from build123d import *

# Parameters (mm, degrees)
SKETCH_1_R          = 65
SKETCH_1_R_2        = 50.2
SKETCH_1_R_3        = 0.5
EXTRUDE_1_DEPTH     = 10
SKETCH_2_R          = 53
CUT_EXTRUDE_1_DEPTH = 8
CUT_EXTRUDE_START   = -8
SKETCH_9_R          = 65
SKETCH_9_R_2        = 55
CUT_EXTRUDE_2_DEPTH = 8
SKETCH_11_R         = 65
SKETCH_11_R_2       = 55
CUT_EXTRUDE_4_DEPTH = 15
SKETCH_12_R         = 53
CUT_EXTRUDE_6_DEPTH = 15
SKETCH_13_R         = 55
SKETCH_13_R_2       = 50.2
EXTRUDE_2_DEPTH     = 2
EXTRUDE_START       = -2
SKETCH_14_R         = 65
SKETCH_14_R_2       = 2.05
SKETCH_14_R_3       = 50.2
EXTRUDE_3_DEPTH     = 2


with BuildPart() as part:
    # 草图1 → 凸台-拉伸1 (new body)
    with BuildSketch(Plane.XY):
        Circle(SKETCH_1_R)
        Circle(SKETCH_1_R_2, mode=Mode.SUBTRACT)
        with Locations((0, 59)):
            Circle(SKETCH_1_R_3, mode=Mode.SUBTRACT)
        with Locations((29.5, 51.095498823)):
            Circle(SKETCH_1_R_3, mode=Mode.SUBTRACT)
        with Locations((51.095498823, 29.5)):
            Circle(SKETCH_1_R_3, mode=Mode.SUBTRACT)
        with Locations((59, 0)):
            Circle(SKETCH_1_R_3, mode=Mode.SUBTRACT)
        with Locations((51.095498823, -29.5)):
            Circle(SKETCH_1_R_3, mode=Mode.SUBTRACT)
        with Locations((29.5, -51.095498823)):
            Circle(SKETCH_1_R_3, mode=Mode.SUBTRACT)
        with Locations((0, -59)):
            Circle(SKETCH_1_R_3, mode=Mode.SUBTRACT)
        with Locations((-29.5, -51.095498823)):
            Circle(SKETCH_1_R_3, mode=Mode.SUBTRACT)
        with Locations((-51.095498823, -29.5)):
            Circle(SKETCH_1_R_3, mode=Mode.SUBTRACT)
        with Locations((-59, 0)):
            Circle(SKETCH_1_R_3, mode=Mode.SUBTRACT)
        with Locations((-51.095498823, 29.5)):
            Circle(SKETCH_1_R_3, mode=Mode.SUBTRACT)
        with Locations((-29.5, 51.095498823)):
            Circle(SKETCH_1_R_3, mode=Mode.SUBTRACT)
    extrude(amount=EXTRUDE_1_DEPTH)

    # 草图2 → 切除-拉伸1 (cut)
    with BuildSketch(Plane(origin=(0, 0, 0), x_dir=(-1, 0, 0), z_dir=(0, 0, -1))):
        Circle(SKETCH_2_R)
    extrude(amount=-CUT_EXTRUDE_1_DEPTH, mode=Mode.SUBTRACT)

    # 草图9 → 切除-拉伸2 (cut)
    with BuildSketch(Plane.XY.offset(10).offset(CUT_EXTRUDE_START)):
        Circle(SKETCH_9_R)
        Circle(SKETCH_9_R_2, mode=Mode.SUBTRACT)
    extrude(amount=CUT_EXTRUDE_2_DEPTH, mode=Mode.SUBTRACT)

    # 草图11 → 切除-拉伸4 (cut, symmetric)
    with BuildSketch(Plane.XY.offset(2)):
        Circle(SKETCH_11_R)
        Circle(SKETCH_11_R_2, mode=Mode.SUBTRACT)
    extrude(amount=CUT_EXTRUDE_4_DEPTH, both=True, mode=Mode.SUBTRACT)

    # 草图12 → 切除-拉伸6 (cut, symmetric)
    with BuildSketch(Plane(origin=(0, 0, 8), x_dir=(-1, 0, 0), z_dir=(0, 0, -1))):
        Circle(SKETCH_12_R)
    extrude(amount=CUT_EXTRUDE_6_DEPTH, both=True, mode=Mode.SUBTRACT)

    # 草图13 → 凸台-拉伸2 (add, symmetric)
    with BuildSketch(Plane(origin=(0, 0, 0), x_dir=(-1, 0, 0), z_dir=(0, 0, -1))):
        with Locations(Location((0, 0, 0), (0, 0, 180))):
            Circle(SKETCH_13_R)
        Circle(SKETCH_13_R_2, mode=Mode.SUBTRACT)
    extrude(amount=EXTRUDE_2_DEPTH, both=True)

    # 草图14 → 凸台-拉伸3 (add)
    with BuildSketch(Plane(origin=(0, 0, -2), x_dir=(-1, 0, 0), z_dir=(0, 0, -1)).offset(EXTRUDE_START)):
        Circle(SKETCH_14_R)
        with Locations((22.57832251, 54.508892418)):
            Circle(SKETCH_14_R_2, mode=Mode.SUBTRACT)
        with Locations((22.57832251, -54.508892418)):
            Circle(SKETCH_14_R_2, mode=Mode.SUBTRACT)
        with Locations((-22.57832251, -54.508892418)):
            Circle(SKETCH_14_R_2, mode=Mode.SUBTRACT)
        with Locations((-22.57832251, 54.508892418)):
            Circle(SKETCH_14_R_2, mode=Mode.SUBTRACT)
        Circle(SKETCH_14_R_3, mode=Mode.SUBTRACT)
        with Locations((-56.344919913, 17.5)):
            Circle(SKETCH_14_R_2, mode=Mode.SUBTRACT)
        with Locations((-56.344919913, -17.5)):
            Circle(SKETCH_14_R_2, mode=Mode.SUBTRACT)
        with Locations((56.344919913, 17.5)):
            Circle(SKETCH_14_R_2, mode=Mode.SUBTRACT)
        with Locations((56.344919913, -17.5)):
            Circle(SKETCH_14_R_2, mode=Mode.SUBTRACT)
    extrude(amount=EXTRUDE_3_DEPTH)


solid = part.part
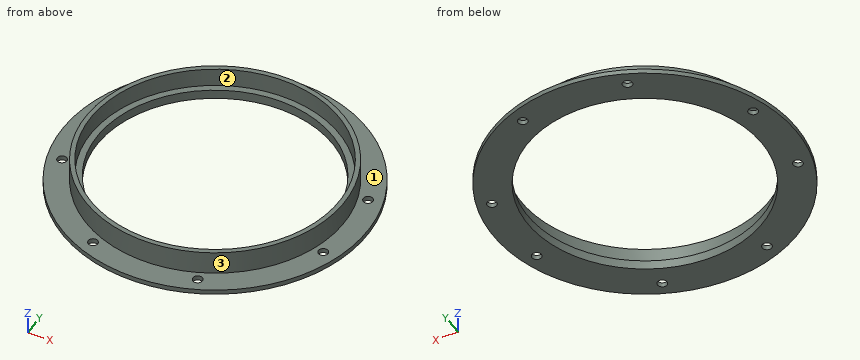
Geometry check sheet. Reference: the model listing, model coordinates, mm. Face numbers are marked on the shaded views. Coordinates: 2 decimals unless noted, no trailing zeros. Order: outer loops, then holes, each group sorted by start corner. A loop starts at its lowest first (then second) coordinate and runs counter-clockwise, first axis right, second up. Notation, with made-up numbers: (-5, 49) - (45, 49) arc R14 cw to (45, 75) - close; hole circle Ø6 at (27.25, -26.75). An arc over 180 degrees is marked (long way). Answer in a Markdown table with one row per item. Add a question column.
1) Cross-section at A-A, the plane y = 0. Record the cut outline in (x, z).
2) Release check for a two-part mould opening along Y. For the marked faces 1, 2 and 3 record: +Y half, -Y half, draft (parallel to the pull), parting line (faces both ways), or undercut.
3) Cross-section at C-C, the plane y = -17.5. Record the cut outline in (x, z), then the cut area to 4 significant figures.
4) Material ranges on line 1 along X through (y, z) = (-1.5, 3); line 2 along Z through (x, y) = (39.5, -44.5); line 3 along Z through (x, y) = (42.5, -31.5), recorded low to high. Write a range as [from, to].
5) Cross-section at D-D, the plane z = 8.5. Record the cut outline in (x, y).
6) Gauge pin test, flat ends, axial feed: P1, Ø5.5, axis at x = -56.34, y = -17.5, coming from the +Z side; P2, Ø2, axis at x = -7.5, z = 8.5, coming from the -Y side; P3, Ø5, axis at x = 41.5, z = -0.5, coming from the +Y side. Record the tip position at first contact, or that the pin passes through.
Check result:
| question | item | result |
|---|---|---|
| 1 | outline | (-65, -2) - (-50.2, -2) - (-50.2, 2) - (-53, 2) - (-53, 10) - (-55, 10) - (-55, 0) - (-65, 0) - close; (50.2, -2) - (65, -2) - (65, 0) - (55, 0) - (55, 10) - (53, 10) - (53, 2) - (50.2, 2) - close |
| 2 | face 1 | draft |
| 2 | face 2 | undercut |
| 2 | face 3 | parting line |
| 3 | outline | (-62.6, -2) - (-58.39, -2) - (-58.39, 0) - (-62.6, 0) - close; (-54.29, -2) - (-47.05, -2) - (-47.05, 2) - (-50.03, 2) - (-50.03, 10) - (-52.14, 10) - (-52.14, 0) - (-54.29, 0) - close; (47.05, -2) - (54.29, -2) - (54.29, 0) - (52.14, 0) - (52.14, 10) - (50.03, 10) - (50.03, 2) - (47.05, 2) - close; (58.39, -2) - (62.6, -2) - (62.6, 0) - (58.39, 0) - close |
| 3 | area | 100.0 mm² |
| 4 | line 1 | x = [-54.98, -52.98], [52.98, 54.98] |
| 4 | line 2 | z = [-2, 0] |
| 4 | line 3 | z = [-2, 2] |
| 5 | outline | circle Ø110 at (0, 0); hole circle Ø106 at (0, 0) |
| 6 | P1 | stops at z = 0 |
| 6 | P2 | stops at y = -54.61 |
| 6 | P3 | stops at y = 52 |
